Geometry: final body of the model. Coordinates: model frame, mm. A direction names the side the tool comes from. Give positions to 0.01 mm unless a question says otherwise; leave off trailing zeros.
1. First-contact query: P1, Ø10, axis at x = 13, z = -154, coming from the -Y side; P2, Ø12, axis at x = 12, z = 150, coming from the +Y side; P3, Ø8, axis at y = 0, z = -266, coming from the +X side; P4, Ø12.5, axis at y = 0, z = -266, coming from the +X side. Flat tips, straight axial feed; report the tip coordinate or a pass-through.
2. Access query for faces 1 (the face through (12, 14, 155)), 2 (the face through (20.056, 2.103, -259.323)), 3 (the face through (9.9, -14, -154.3)). Directions: +Z, -Z, +X, -X, +Y, -Y. A direction counts if a zero-diameter tool reaches every point of the face in a straight line with its end or side. Return the directions, or none.
3. Draft query along Z for faces 4 (the face through (12, 0, -341)), 5 (the face through (24, 0, 5)), 6 (the face through (12, 0, 341)), 7 (the face through (16, 0, -261)). Return one class per face: +Z half, -Z half, draft (parallel to the pull), parting line (faces both ways), or undercut.
4. Material intervals for line 1 along Y through (x, z) = (2, -266.5); line 2 along Z through (x, y) = (6.75, -16.5); line 3 along X through (y, z) = (16, -150), sorted ascending.
5. Section A-A, the plane x = 12. State how many separate pieces and enclosed holes the cut face has, then the cut area to 3 significant figures.
from build123d import *

# Parameters (mm, degrees)
ESQUISSE1_W             = 682
ESQUISSE1_H             = 48
BOSS_EXTRU_1_DEPTH      = 24
ESQUISSE2_R             = 4.5
ENL_V_MAT_EXTRU_1_DEPTH = 346.197045179
ESQUISSE3_R             = 10
ENL_V_MAT_EXTRU_2_DEPTH = 10
ESQUISSE4_R             = 7
ENL_V_MAT_EXTRU_3_DEPTH = 10
ESQUISSE5_R             = 1.5
ENL_V_MAT_EXTRU_4_DEPTH = 343.68498654
ESQUISSE6_R             = 4.5
ENL_V_MAT_EXTRU_5_DEPTH = 343.68498654
ESQUISSE7_R             = 7
ENL_V_MAT_EXTRU_6_DEPTH = 8


with BuildPart() as part:
    # Esquisse1 → Boss.-Extru.1 (new body)
    with BuildSketch(Plane(origin=(0, 0, 0), x_dir=(0, 0, -1), z_dir=(1, 0, 0))):
        Rectangle(ESQUISSE1_W, ESQUISSE1_H)
    extrude(amount=BOSS_EXTRU_1_DEPTH)

    # Esquisse2 → Enlèv. mat.-Extru.1 (cut, through all)
    with BuildSketch(Plane.XZ.offset(24)):
        with Locations(Location((12, 150, 0), (0, 0, 270))):
            Circle(ESQUISSE2_R)
        with Locations(Location((12, -150, 0), (0, 0, 270))):
            Circle(ESQUISSE2_R)
    extrude(amount=-ENL_V_MAT_EXTRU_1_DEPTH, mode=Mode.SUBTRACT)

    # Esquisse3 → Enlèv. mat.-Extru.2 (cut)
    with BuildSketch(Plane.XZ.offset(24)):
        with Locations(Location((12, 150, 0), (0, 0, 270))):
            Circle(ESQUISSE3_R)
        with Locations(Location((12, -150, 0), (0, 0, 270))):
            Circle(ESQUISSE3_R)
    extrude(amount=-ENL_V_MAT_EXTRU_2_DEPTH, mode=Mode.SUBTRACT)

    # Esquisse4 → Enlèv. mat.-Extru.3 (cut)
    with BuildSketch(Plane(origin=(0, 24, 0), x_dir=(-1, 0, 0), z_dir=(0, 1, 0))):
        with Locations(Location((-12, 150, 0), (0, 0, 90))):
            Circle(ESQUISSE4_R)
        with Locations(Location((-12, -150, 0), (0, 0, 90))):
            Circle(ESQUISSE4_R)
    extrude(amount=-ENL_V_MAT_EXTRU_3_DEPTH, mode=Mode.SUBTRACT)

    # Esquisse5 → Enlèv. mat.-Extru.4 (cut, through all)
    with BuildSketch(Plane(origin=(24, 0, 0), x_dir=(0, 0, -1), z_dir=(1, 0, 0))):
        with Locations((-216, 0)):
            Circle(ESQUISSE5_R)
    extrude(amount=-ENL_V_MAT_EXTRU_4_DEPTH, mode=Mode.SUBTRACT)

    # Esquisse6 → Enlèv. mat.-Extru.5 (cut, through all)
    with BuildSketch(Plane.ZY):
        with Locations((-266, 0)):
            Circle(ESQUISSE6_R)
    extrude(amount=-ENL_V_MAT_EXTRU_5_DEPTH, mode=Mode.SUBTRACT)

    # Esquisse7 → Enlèv. mat.-Extru.6 (cut)
    with BuildSketch(Plane.ZY.offset(-24)):
        with Locations((-266, 0)):
            Circle(ESQUISSE7_R)
    extrude(amount=ENL_V_MAT_EXTRU_6_DEPTH, mode=Mode.SUBTRACT)


solid = part.part
Answers below:
1. P1: stops at y = -14
1. P2: stops at y = 14
1. P3: passes through
1. P4: stops at x = 16
2. face 1: +Y
2. face 2: +X
2. face 3: -Y
3. face 4: -Z half
3. face 5: draft
3. face 6: +Z half
3. face 7: undercut
4. line 1: y = -24 to -4.47, 4.47 to 24
4. line 2: z = -341 to -158.51, -141.49 to 141.49, 158.51 to 341
4. line 3: x = 0 to 5, 19 to 24
5. separate pieces: 3
5. enclosed holes: 2
5. area: 31,500 mm2
